For this review, take the finished solid that the model builds, in its own axes (mm). Face numbers are marked on the shaded views. Give positions to 0.01 mm unless a question says otherwise; leave off trailing zeros. Write each loop counter-clockwise with the first axis right and the second up, starting at its lowest first coordinate (ties: lowest second). Pieces come first, ordered by that corner, then holes. Notation, with made-up numbers: M 64.25,72 L 109.25,72 A24 cw 109.25,87 Z; hole C 87.25,29 d4. An arc over 180 degrees is marked long. One line per item, written item: value. Start each with the question number.
Item 1: Mouldability with a two-part tool opening along Z and no side actions: class the marked faces 1, 2 and 3 as released by +Z, released by -Z, zero draft, split by the parting line, or undercut.
Item 2: To check wall thickness, follow probe 1 along Y at (x, z) = (36, -158); probe 2 along X at (y, z) = (28, -97); probe 3 along Z at (x, y) = (112.5, 28). State the ranges of each line that lie inside material, in increasing order.
Item 3: Consider section B-B, the plane y = 38.5. Write out the cut boundary in (x, z) (3 decimals), and give its area (3 significant figures).
Item 4: Consider section A-A, the plane y = 19.5. Write out the cut boundary in (x, z) (3 decimals).
Item 5: Clearance check with flat-ended pins moving along their axes: pin 1 Ø1.1 at (x, z) = (111, -123.5) entering from -Y; pin 2 Ø25 at (x, z) = (54, -139) entering from +Y; pin 3 Ø6.5 at (x, z) = (6.35, -157.54) entering from +Y; pin 4 Ø5 at (y, z) = (13, -111.5) entering from -X. State where each tip first meets the part, or that it passes through.
```python
from build123d import *

# Parameters (mm, degrees)
BOSS_EXTRUDE1_DEPTH        = 6.35
BOSS_EXTRUDE2_DEPTH        = 44.45
CUT_EXTRUDE1_DEPTH         = 34.29
F_10_32_TAPPED_HOLE1_D     = 4.0386
F_10_32_TAPPED_HOLE1_DEPTH = 6.35
BOSS_EXTRUDE3_DEPTH        = 3.175
CIRPATTERN1_COUNT          = 2
CIRPATTERN1_ANGLE          = 47.375
FILLET1_R                  = 4.7625


with BuildPart() as part:
    # Sketch1 → Boss-Extrude1 (new body)
    with BuildSketch(Plane(origin=(0, 0, 0), x_dir=(1, 0, 0), z_dir=(0, 1, 0))):
        with BuildLine():
            Line((165.608, 0), (146.558, 0))
            ThreePointArc((146.558, 0), (103.632155637, -103.632155637), (0, -146.558))
            Line((0, -146.558), (0, -165.608))
            ThreePointArc((0, -165.608), (117.102539819, -117.102539819), (165.608, 0))
        make_face()
    extrude(amount=BOSS_EXTRUDE1_DEPTH)

    # Sketch2 → Boss-Extrude2 (add)
    with BuildSketch(Plane(origin=(0, 6.35, 0), x_dir=(1, 0, 0), z_dir=(0, 1, 0))):
        with BuildLine():
            Line((146.558, 0), (149.733, 0))
            ThreePointArc((149.733, 0), (105.877219667, -105.877219667), (0, -149.733))
            Line((0, -149.733), (0, -146.558))
            ThreePointArc((0, -146.558), (103.632155637, -103.632155637), (146.558, 0))
        make_face()
    extrude(amount=BOSS_EXTRUDE2_DEPTH)

    # Sketch3 → Cut-Extrude1 (cut)
    with BuildSketch(Plane(origin=(0, 50.8, 0), x_dir=(1, 0, 0), z_dir=(0, 1, 0))):
        with BuildLine():
            Line((96.677867382, -110.148251563), (98.927586748, -112.39797093))
            ThreePointArc((98.927586748, -112.39797093), (52.869111529, -140.088644562), (0, -149.733))
            Line((0, -149.733), (0, -146.558))
            ThreePointArc((0, -146.558), (51.65336345, -137.153845766), (96.677867382, -110.148251563))
        make_face()
    extrude(amount=-CUT_EXTRUDE1_DEPTH, mode=Mode.SUBTRACT)

    # #10-32 Tapped Hole1
    with Locations(Plane(origin=(0, 6.35, 0), x_dir=(1, 0, 0), z_dir=(0, 1, 0))):
        with Locations((6.35, -157.542578595), (87.858258413, -130.923309609), (143.383000088, -65.58431105)):
            Hole(F_10_32_TAPPED_HOLE1_D / 2, depth=F_10_32_TAPPED_HOLE1_DEPTH)

    # Sketch9 → Boss-Extrude3 (add)
    with BuildSketch(Plane(origin=(0, 0, 0), x_dir=(-1, 0, 0), z_dir=(0, 0, -1))):
        Polygon((-165.608, 6.35), (-149.733, 50.8), (-146.558, 50.8), (-146.558, 6.35), align=None)
    boss_extrude3 = extrude(amount=-BOSS_EXTRUDE3_DEPTH)

    # CirPattern1: Boss-Extrude3 ×2 about axis
    cirpattern1_axis = Axis((0, 0, 0), (0, -1, 0))
    for i in range(1, CIRPATTERN1_COUNT):
        add(boss_extrude3.rotate(cirpattern1_axis, i * CIRPATTERN1_ANGLE / (CIRPATTERN1_COUNT - 1)))

    # Fillet1
    fillet1_edges = [part.edges().sort_by_distance(p)[0] for p in [
        (52.939054251, 6.35, 140.062228399),
        (136.472515739, 6.35, 61.605387238),
    ]]
    fillet(fillet1_edges, radius=FILLET1_R)


with BuildPart() as body_2:
    # Mirror1: mirrored copy
    add(part.part.mirror(Plane.XY))


solid = body_2.part
```
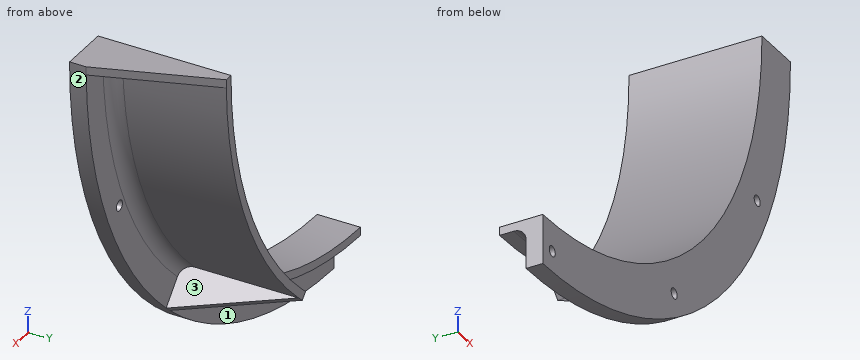
Model answer:
1. face 1: zero draft
1. face 2: released by -Z
1. face 3: undercut
2. probe 1: y = 0 to 6.35
2. probe 2: x = 109.86 to 114.07
2. probe 3: z = -98.81 to -93.93
3. outline: M 96.678,-110.148 L 98.928,-112.398 A149.733 ccw 99.04,-112.299 L 102.037,-115.556 L 104.374,-113.406 L 101.399,-110.174 A149.733 ccw 149.699,-3.175 L 154.126,-3.175 L 154.126,0 L 146.558,0 A146.558 cw Z
3. area: 428 mm2
4. outline: M 96.678,-110.148 L 98.928,-112.398 A149.733 ccw 99.04,-112.299 L 106.633,-120.549 L 108.969,-118.399 L 101.399,-110.174 A149.733 ccw 149.699,-3.175 L 160.912,-3.175 L 160.912,0 L 146.558,0 A146.558 cw Z
5. pin 1: stops at y = 0
5. pin 2: stops at y = 16.51
5. pin 3: stops at y = 6.35
5. pin 4: stops at x = 92.1
